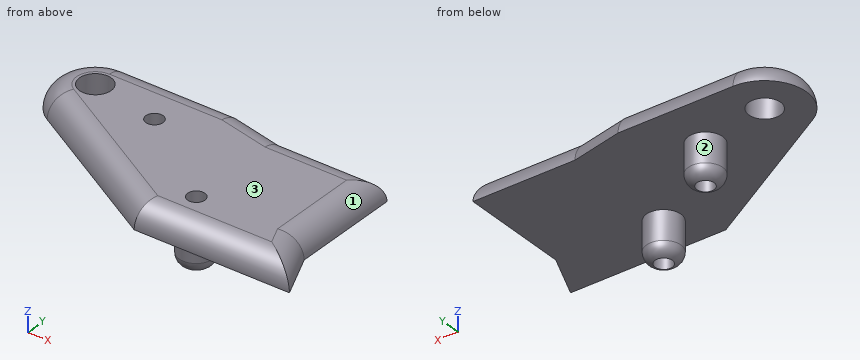
from build123d import *

# Parameters (mm, degrees)
F0_R     = 3
F0_R_2   = 2.75
F0_R_3   = 1.5
F1_DEPTH = 4
F2_DEPTH = 7
F4_R     = 3.99999


# Not quite as in the source:
# - a fillet or chamfer that OpenCascade refuses, or shapes differently, is made with other operations: its cross-section is extruded or revolved along the edge and cut away or added
# - a fillet or chamfer is up to 0.001 mm smaller than in the source, because OpenCascade refuses the exact size


with BuildPart() as f1:
    # F0 (on Top) → F1 (new body)
    with BuildSketch(Plane.XY):
        with BuildLine():
            Line((0, 0), (23.5013441249, 0))
            Line((23.5013441249, 0), (23.5013441249, 8))
            Line((23.5013441249, 8), (23.5013441249, 27))
            Line((23.5013441249, 27), (5.7513441249, 27))
            Line((5.7513441249, 27), (-3.2486558751, 29))
            Line((-3.2486558751, 29), (-23.2486558751, 29))
            ThreePointArc((-23.2486558751, 29), (-30.2527750248, 23.6221150973), (-26.8659020001, 15.4668455))
            Line((-26.8659020001, 15.4668455), (0, 0))
        make_face()
        with Locations((5.5013441249, 7)):
            Circle(F0_R, mode=Mode.SUBTRACT)
        with Locations((-23.2486558751, 21.75)):
            Circle(F0_R_2, mode=Mode.SUBTRACT)
        with Locations((-11.2486558751, 19.5)):
            Circle(F0_R, mode=Mode.SUBTRACT)
        Polygon((23.5013441249, 8), (23.5013441249, 0), (27.0013441249, 0), align=None)
        with Locations((-11.2486558751, 19.5)):
            Circle(F0_R)
        with Locations((-11.2486558751, 19.5)):
            Circle(F0_R_3, mode=Mode.SUBTRACT)
        with Locations((5.5013441249, 7)):
            Circle(F0_R)
        with Locations((5.5013441249, 7)):
            Circle(F0_R_3, mode=Mode.SUBTRACT)
    extrude(amount=F1_DEPTH)

    # F0 (on Top) → F2 (join)
    with BuildSketch(Plane.XY):
        with Locations((-11.2486558751, 19.5)):
            Circle(F0_R)
        with Locations((-11.2486558751, 19.5)):
            Circle(F0_R_3, mode=Mode.SUBTRACT)
        with Locations((5.5013441249, 7)):
            Circle(F0_R)
        with Locations((5.5013441249, 7)):
            Circle(F0_R_3, mode=Mode.SUBTRACT)
    extrude(amount=-F2_DEPTH)

    # F3: fillet of radius 2 on 2 edges, made by hand

    # F3_s1 → F3_t2 (revolve, cut)
    with BuildSketch(Plane.XZ.offset(-19.5)):
        with BuildLine():
            ThreePointArc((-9.7486558751, -7), (-8.667517045, -6.2882531983), (-8.2486558751, -5.0635083269))
            Line((-8.2486558751, -5.0635083269), (-8.2486558751, -7))
            Line((-8.2486558751, -7), (-9.7486558751, -7))
        make_face()
    revolve(axis=Axis((-11.2486558751, 19.5, -7), (0, 0, 1)), mode=Mode.SUBTRACT)

    # F3_s3 → F3_t4 (revolve, cut)
    with BuildSketch(Plane.XZ.offset(-7)):
        with BuildLine():
            ThreePointArc((7.0013441249, -7), (8.082482955, -6.2882531983), (8.5013441249, -5.0635083269))
            Line((8.5013441249, -5.0635083269), (8.5013441249, -7))
            Line((8.5013441249, -7), (7.0013441249, -7))
        make_face()
    revolve(axis=Axis((5.5013441249, 7, -7), (0, 0, 1)), mode=Mode.SUBTRACT)

    # F4 (radius 4 in the source; OpenCascade refuses exactly that, so slightly less here)
    f4_edges = [f1.edges().sort_by_distance(p)[0] for p in [
        (-13.248656, 29, 4),
        (13.500672, 0, 4),
        (25.251344, 4, 4),
        (23.501344, 17.5, 4),
        (1.251344, 28, 4),
        (14.626344, 27, 4),
        (-13.432951, 7.733423, 4),
        (-30.252775, 23.622115, 4),
    ]]
    fillet(f4_edges, radius=F4_R)


solid = f1.part
Verification items for the finished model (mm, model axes). Face numbers are marked on the shaded views. A direction names the side the tool comes from. Round coordinates to 2 decimals unless told otherwise and drop trailing zeros. Order: outer loops, then holes, each group sorted by start corner. A loop starts at its lowest first (then second) coordinate and runs counter-clockwise, first axis right, second up. Notation, with made-up numbers: (-40, 33) -> (-11, 33) arc R29 cw to (-11, 68) -> close; hole circle Ø3 at (34.25, 51.5). An arc over 180 degrees is marked (long way). Put each result on its own line as item: value.
1) Set-up check for the marked faces 1, 2 and 3: record each of +Z, -Z, +X, -X, +Y, -Y from which the full face is reachable in a straight line by a thin tool's end or side.
Final values:
face 1: +Z, +X, +Y
face 2: -Z
face 3: +Z, +X, -X, +Y, -Y
2) Section check A-A (z = -2.75). Record the cut outline in (x, y).
Final values:
outline: circle Ø6 at (-11.25, 19.5); circle Ø6 at (5.5, 7); hole circle Ø3 at (-11.25, 19.5); hole circle Ø3 at (5.5, 7)
3) Material ranges on line 1 (Z direction, x = 1, y = 22); line 2 (X direction, y = 7.5, z = -2.75); line 3 (X direction, y = 20.25, z = -5.5), recorded low to high.
Final values:
line 1: z = 0 to 4
line 2: x = 2.54 to 4.09, 6.92 to 8.46
line 3: x = -14.1 to -12.55, -9.95 to -8.39
4) Depth check by flat-ended pin: pin 1 (3.5 mm diameter, centred on x = 5.5, y = 7, fed in from -Z); pin 2 (1 mm diameter, centred on y = 15, z = -1.5, fed in from -X); pin 3 (4 mm diameter, centred on y = 22, z = -2.5, fed in from -X); pin 4 (3 mm diameter, centred on x = 7, z = 1.5, fed in from +Y). Enter the tip coordinate at first touch or a pass-through.
Final values:
pin 1: stops at z = -7
pin 2: passes through
pin 3: stops at x = -14.21
pin 4: stops at y = 27
